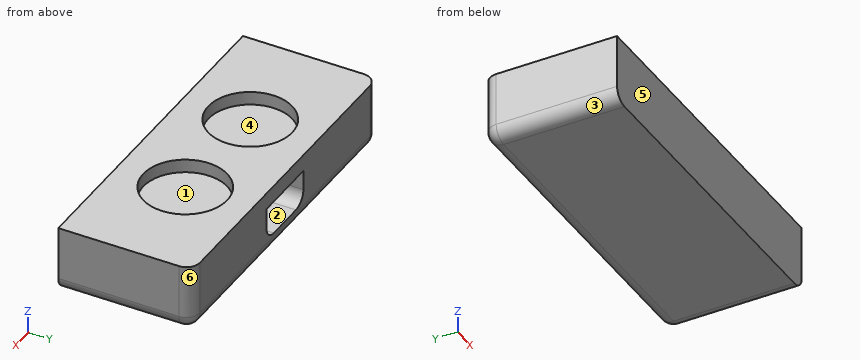
Autodesk Inventor part; units mm, degrees
ref_plane "YZ Plane" through (0, 0, 0) normal (1, 0, 0) x (0, 1, 0)
ref_plane "XZ Plane" through (0, 0, 0) normal (0, 1, 0) x (-1, 0, 0)
ref_plane "XY Plane" through (0, 0, 0) normal (0, 0, 1) x (1, 0, 0)
sketch "Sketch6" plane through (0, 0, 0) normal (0, 0, 1) x (1, 0, 0)
  line L0 (0, 0) -> (-50, 0)
  line L1 (-50, 0) -> (-50, 20)
  line L2 (-50, 20) -> (0, 20)
  line L3 (0, 20) -> (0, 0)
  dimension "d55" = 50
  dimension "d56" = 20
extrude "Extrusion5" add sketch "Sketch6" along normal blind 10
sketch "Sketch7" plane through (0, 0, 10) normal (0, 0, 1) x (1, 0, 0)
  circle A0 centre (-33.8, 10) radius 6.25
  circle A1 centre (-16.2, 10) radius 6.25
  point P0 (0, 0)
  dimension "d59" = 12.5
  dimension "d60" = 12.5
extrude "Extrusion6" cut sketch "Sketch7" against normal blind 2
sketch "Sketch8" plane through (-50, 20, 0) normal (0, 1, 0) x (1, 0, 0)
  line L0 (50, 0) -> (30, 0)
  line L1 (30, 0) -> (30, -2.5)
  line L2 (30, -2.5) -> (50, -2.5)
  line L3 (50, -2.5) -> (50, 0)
  line L4 (30, -2.5) -> (20, -2.5)
  line L5 (20, -2.5) -> (20, -7.5)
  line L6 (20, -7.5) -> (30, -7.5)
  line L7 (30, -7.5) -> (30, -2.5)
  dimension "d63" = 20
  dimension "d64" = 2.5
  dimension "d65" = 10
  dimension "d66" = 5
extrude "Extrusion7" cut sketch "Sketch8" against normal blind 10 contours L7 L6 L5 L4
fillet "Fillet4" radius 2 2 edges at (-30, 15, 2.5) (-20, 15, 2.5)
fillet "Fillet5" radius 2 5 edges at (0, 20, 5) (-50, 20, 5) (-50, 10, 0) (-25, 20, 0) (0, 10, 0)
properties part number "A1 Holder"
CAD build for the part. Positions are in the model's coordinates, mm. Face numbers are marked on the shaded views. A direction names the side the tool comes from. Round coordinates to 2 decimals unless told otherwise and drop trailing zeros. Order: outer loops, then holes, each group sorted by start corner. A loop starts at its lowest first (then second) coordinate and runs counter-clockwise, first axis right, second up. Notation, with made-up numbers: (-24, -22) -> (-19, -22) arc R23 cw to (-19, 13) -> close; hole circle Ø10 at (9, 55.5). An arc over 180 degrees is marked (long way). Write item = value, one per line.
(1) Pull direction Y, two halves, no side cores. Call the marked faces 4, 5 and 6: +Y half, -Y half, draft (parallel to the pull), parting line (faces both ways), or undercut.
Answers follow:
face_4 = undercut
face_5 = -Y half
face_6 = +Y half
(2) Flat gauge pins, fed straight in: P1, Ø1, axis at x = -45, z = 3, coming from the -Y side; P2, Ø4, axis at x = -18.5, y = 12, coming from the +Z side. Where does each tip first touch, or does it go through?
Answers follow:
P1 = 0
P2 = 8
(3) Drill centre lines: L1, parallel to Z at x = -20, y = 6; L2, parallel to Y at x = -16.2, z = 9.6; L3, parallel to X at y = 4.25, z = 9.25. Where is each one in solid material? Low to high.
Answers follow:
L1 = 0 to 8
L2 = 0 to 3.75, 16.25 to 20
L3 = -50 to -36.25, -31.35 to -18.65, -13.75 to 0
(4) Cut at B-B (x = -16.2). Write the cut outline in (y, z), plus the area to 3 significant figures.
Answers follow:
outline = (0, 0) -> (18, 0) arc R2 ccw to (20, 2) -> (20, 10) -> (16.25, 10) -> (16.25, 8) -> (3.75, 8) -> (3.75, 10) -> (0, 10) -> close
area = 174 mm²
(5) 3-axis set-ups, long thin cutter, end or side, ignore diameter. For the marked faces 1, 2 and 3: which of +Z, -Z, +X, -X, +Y, -Y reach the whole face in a straight line?
Answers follow:
face_1 = +Z
face_2 = +Y
face_3 = -Z, -X, +Y, -Y
(6) Cut at D-D (y = 18.75). Write the cut outline in (x, z).
Answers follow:
outline = (-49.85, 2) arc R1.85 ccw to (-48, 0.15) -> (-2, 0.15) arc R1.85 ccw to (-0.15, 2) -> (-0.15, 10) -> (-49.85, 10) -> close; hole (-30, 4.5) arc R2 ccw to (-28, 2.5) -> (-22, 2.5) arc R2 ccw to (-20, 4.5) -> (-20, 7.5) -> (-30, 7.5) -> close
(7) Cut at C-C (z = 6.5). Write the cut outline in (x, y), plus the area to 3 significant figures.
Answers follow:
outline = (-50, 0) -> (0, 0) -> (0, 18) arc R2 ccw to (-2, 20) -> (-20, 20) -> (-20, 10) -> (-30, 10) -> (-30, 20) -> (-48, 20) arc R2 ccw to (-50, 18) -> close
area = 898 mm²
(8) Cut at A-A (y = 16.75). Write the cut outline in (x, z), plus the area to 3 significant figures.
Answers follow:
outline = (-50, 2) arc R2 ccw to (-48, 0) -> (-2, 0) arc R2 ccw to (0, 2) -> (0, 10) -> (-50, 10) -> close; hole (-30, 4.5) arc R2 ccw to (-28, 2.5) -> (-22, 2.5) arc R2 ccw to (-20, 4.5) -> (-20, 7.5) -> (-30, 7.5) -> close
area = 450 mm²
